Can you work these out from the model? Positions are in its coordinate system, mm. Face numbers are marked on the shaded views. Round coordinates to 2 decimals unless told otherwise and drop trailing zeros. Order: outer loops, then holes, each group sorted by start corner. A loop starts at its lowest first (then second) coordinate and runs counter-clockwise, first axis right, second up. Notation, with made-up numbers: M -16,6 L 39,6 A23 ccw 39,16 Z; hole C -21.5,-15.5 d11. An arc over 180 degrees is marked long. One line per question, with ' | ' between items.
```python
from build123d import *

# Parameters (mm, degrees)
F1_DEPTH = 270
F3_DEPTH = 250


with BuildPart() as f1:
    # F0 (on Top) → F1 (new body, symmetric)
    with BuildSketch(Plane.XY):
        with BuildLine():
            Line((79.9999999672, 79.9977099118), (80.0017351981, 140.6147968648))
            Line((80.0017351981, 140.6147968648), (75.0017352002, 140.6149399953))
            Line((75.0017352002, 140.6149399953), (74.9999999686, 79.9978290345))
            ThreePointArc((74.9999999686, 79.9978290345), (-0.0021469583, 4.9999760229), (-74.99999997, 80.0021229498))
            Line((-74.99999997, 80.0021229498), (-74.9982647384, 140.6192339106))
            Line((-74.9982647384, 140.6192339106), (-79.9982647363, 140.6193770411))
            Line((-79.9982647363, 140.6193770411), (-79.9999999672, 80.0022900882))
            ThreePointArc((-79.9999999672, 80.0022900882), (-0.0022900882, 3.28e-08), (79.9999999672, 79.9977099118))
        make_face()
    extrude(amount=F1_DEPTH, both=True)

    # F2 (on Right) → F3 (cut, symmetric)
    with BuildSketch(Plane.YZ):
        with BuildLine():
            Line((140.6193770411, -270), (140.6193770411, 270))
            Line((140.6193770411, 270), (0, 270))
            Line((0, 270), (0, 219.99933))
            Line((0, 219.99933), (110.6193770411, 219.99933))
            Line((110.6193770411, 219.99933), (110.6193770411, 115.1882235752))
            Line((110.6193770411, 115.1882235752), (60.6193770411, 5))
            Line((60.6193770411, 5), (10.9110071197, -36.0003965298))
            ThreePointArc((10.9110071197, -36.0003965298), (2.8645086058, -46.3504872547), (0, -59.1436536647))
            Line((0, -59.1436536647), (0, -270))
            Line((0, -270), (140.6193770411, -270))
        make_face()
    extrude(amount=F3_DEPTH, both=True, mode=Mode.SUBTRACT)


solid = f1.part
```
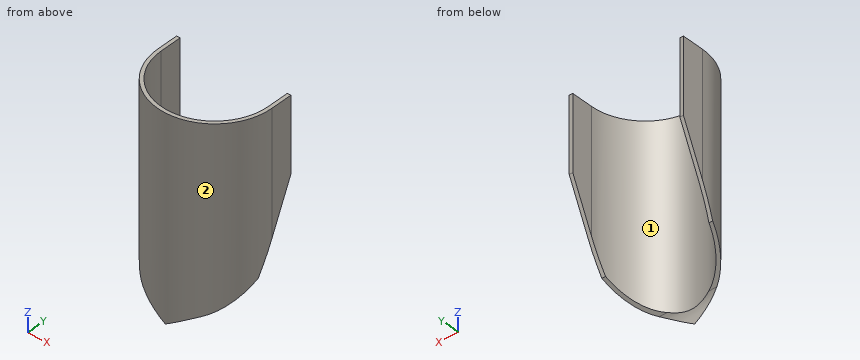
(1) Please list where these lines run through material, in increasing order: probe 1 along X at (y, z) = (82, 89.5); probe 2 along X at (y, z) = (13.5, 12); probe 3 along Y at (x, z) = (12, 113.5). Write a range as [from, to].
Final values:
probe 1: [-80, -75], [75, 80] | probe 2: [-44.47, -34.68], [34.68, 44.47] | probe 3: [0.91, 5.97]
(2) Thinking about a two-plate mould opening in X: for the marked faces 1 and 2, which applies, released by +X, released by -X, zero draft, split by the parting line, or undercut?
Final values:
face 1: undercut | face 2: split by the parting line
(3) If we section it at C-C on y = 103: Please give me the cut outline in (x, z), plus the area to 3 significant figures.
Final values:
outline: M -80,98.4 L -75,98.4 L -75,220 L -80,220 Z; M 75,98.4 L 80,98.4 L 80,220 L 75,220 Z | area: 1,220 mm^2
(4) If we section it at A-A on y = 17.5: Please give me the cut outline in (x, z).
Final values:
outline: M -49.94,-30.57 L -41.46,-30.57 L -41.46,220 L -49.94,220 Z; M 41.46,-30.57 L 49.94,-30.57 L 49.94,220 L 41.46,220 Z
(5) If we section it at D-D on x = 0: Please give me the cut outline in (y, z).
Final values:
outline: M 0,-59.14 A30 cw 5,-42.56 L 5,220 L 0,220 Z
(6) If we section it at B-B on z = 161: Please give me the cut outline in (x, y).
Final values:
outline: M -80,80 A80 ccw 80,80 L 80,110.62 L 75,110.62 L 75,80 A75 cw -75,80 L -75,110.62 L -80,110.62 Z
(7) Will these pins go through, and if not, where does the flat tip stop? pin 1 Ø3 at (x, z) = (61, 88.5) entering from +Y; pin 2 Ø8 at (x, z) = (-44, -27) entering from -Y; pin 3 Ø4 at (x, z) = (2.5, 120) entering from -Y.
Final values:
pin 1: y = 38.54 | pin 2: y = 10.72 | pin 3: y = 0
